Work out the finished part from the listing and answer in its coordinate system (mm). Give positions to 0.01 mm unless a question says otherwise; leave off trailing zeros. Write each loop counter-clockwise with the first axis right and the second up, starting at its lowest first coordinate (ties: lowest second). Pieces come first, ordered by that corner, then holes. Notation, with made-up numbers: (5, 26.25) -> (10, 26.25) arc R23 ccw to (10, 60.25) -> close; hole circle Ø8 at (3, 50.25). An arc over 180 degrees is marked (long way). Use a Markdown table: item, result. Add a question column.
Q1. Section A-A, the plane z = -18.5 is taken. Give the vertices of the cut face in (x, y), plus the area to 3 significant figures.
Q2. Section B-B, the plane y = 3.9 is taken. State how many separate pieces and enclosed holes the cut face has, plus the area to 3 significant figures.
Q3. Each of these flat-tipped pins is pushed along its axis until it touches: pin 1 Ø3 at (x, y) = (-9.5, 2.5) entering from -Z; pin 2 Ø9 at (x, z) = (-15, -115) entering from +Y. Where does it stop, or does it pass through?
Q4. Section D-D, the plane x = -23.5 is taken. Give the vertices of the cut face in (y, z).
Q5. Section C-C, the plane z = -117 is taken. Give the vertices of the cut face in (x, y).
Q6. Consider line 1 (Z direction, x = -15, y = 2.4); line 2 (X direction, y = 1.8, z = -115); line 3 (Z direction, x = -17.5, y = 1.9). Determine where each line is inside the solid, lowest interval first.
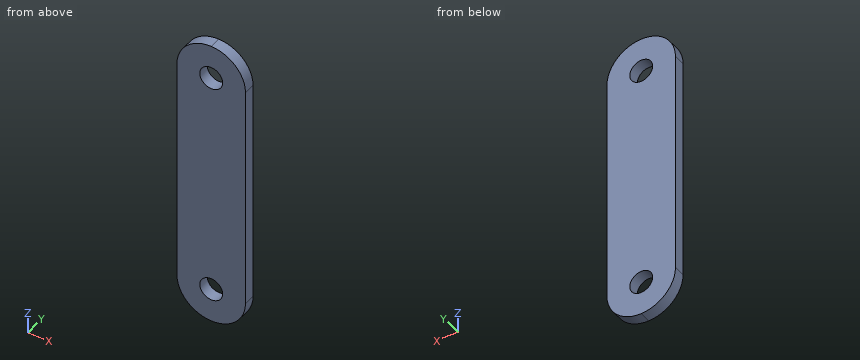
Autodesk Inventor part; units mm, degrees
ref_plane "YZ Plane" through (0, 0, 0) normal (1, 0, 0) x (0, 1, 0)
ref_plane "XZ Plane" through (0, 0, 0) normal (0, 1, 0) x (-1, 0, 0)
ref_plane "XY Plane" through (0, 0, 0) normal (0, 0, 1) x (1, 0, 0)
sketch "Sketch1" plane through (0, 0, 0) normal (0, 1, 0) x (-1, 0, 0)
  line L0 (0, 0) -> (30, 0)
  line L1 (30, 0) -> (30, -130)
  line L2 (30, -130) -> (0, -130)
  line L3 (0, -130) -> (0, 0)
  dimension "d0" = 30
  dimension "d1" = 130
extrude "Extrusion1" add sketch "Sketch1" along normal blind 5
fillet "Fillet1" radius 15 4 edges at (0, 2.5, 0) (-30, 2.5, 0) (0, 2.5, -130) (-30, 2.5, -130)
sketch "Sketch2" plane through (0, 5, 0) normal (0, 1, 0) x (1, 0, 0)
  arc A0 (-30, 15) -> (0, 15) centre (-15, 15) ccw
  circle A1 centre (-15, 15) radius 5
  arc A2 (0, 115) -> (-30, 115) centre (-15, 115) ccw
  circle A3 centre (-15, 115) radius 5
  point P0 (0, 0)
  dimension "d5" = 10
  dimension "d6" = 10
extrude "Extrusion2" cut sketch "Sketch2" against normal blind 10
equation "\"d7\" = d6"
properties part number "Rocker"
Result set:
| question | item | result |
|---|---|---|
| 1 | outline | (-30, 0) -> (-18.57, 0) -> (-18.57, 5) -> (-30, 5) -> close; (-11.43, 0) -> (0, 0) -> (0, 5) -> (-11.43, 5) -> close |
| 1 | area | 114 mm2 |
| 2 | separate pieces | 1 |
| 2 | enclosed holes | 2 |
| 2 | area | 3,550 mm2 |
| 3 | pin 1 | stops at z = -129.46 |
| 3 | pin 2 | passes through |
| 4 | outline | (0, -127.36) -> (5, -127.36) -> (5, -2.64) -> (0, -2.64) -> close |
| 5 | outline | (-29.87, 0) -> (-19.58, 0) -> (-19.58, 5) -> (-29.87, 5) -> close; (-10.42, 0) -> (-0.13, 0) -> (-0.13, 5) -> (-10.42, 5) -> close |
| 6 | line 1 | z = -130 to -120, -110 to -20, -10 to 0 |
| 6 | line 2 | x = -30 to -20, -10 to 0 |
| 6 | line 3 | z = -129.79 to -119.33, -110.67 to -19.33, -10.67 to -0.21 |
